from build123d import *

# Parameters (mm, degrees)
SKETCH046_R     = 2.5
PAD023_DEPTH    = 2.5
SKETCH047_R     = 5
PAD024_DEPTH    = 3
FILLET003_R     = 1.5
SKETCH049_R     = 2.5
PAD025_DEPTH    = 4
SKETCH050_R     = 1.5
POCKET026_DEPTH = 4
PAD056_DEPTH    = 0.2


with BuildPart() as part:
    # Sketch046 → Pad023 (new body)
    with BuildSketch(Plane(origin=(0, 0, 30), x_dir=(1, 0, 0), z_dir=(0, 0, -1))):
        with Locations((101, 55)):
            Circle(SKETCH046_R)
    extrude(amount=-PAD023_DEPTH)

    # Sketch047 (on Face3 of Pad023) → Pad024 (join)
    with BuildSketch(Plane.XY.offset(32.5)):
        with Locations((101, -55)):
            Circle(SKETCH047_R)
    extrude(amount=PAD024_DEPTH)

    # Fillet003
    fillet003_edges = [part.edges().sort_by_distance(p)[0] for p in [
        (96, -55, 35.5),
    ]]
    fillet(fillet003_edges, radius=FILLET003_R)

    # Sketch049 → Pad025 (join)
    with BuildSketch(Plane(origin=(0, 0, 30), x_dir=(1, 0, 0), z_dir=(0, 0, -1))):
        with Locations((101, 55)):
            Circle(SKETCH049_R)
    extrude(amount=PAD025_DEPTH)

    # Sketch050 (on Face17 of Pad025) → Pocket026 (cut)
    with BuildSketch(Plane(origin=(0, 0, 26), x_dir=(1, 0, 0), z_dir=(0, 0, -1))):
        with Locations((101, 55)):
            Circle(SKETCH050_R)
    extrude(amount=-POCKET026_DEPTH, mode=Mode.SUBTRACT)


with BuildPart() as part_1:
    # Body002 placement: moved
    add(part.part.moved(Location((75, 0, 0))))

    # Sketch090 (on Face4 of Clone004) → Pad056 (new body)
    with BuildSketch(Plane(origin=(75, 0, 35.5), x_dir=(1, 0, 0), z_dir=(0, 0, 1))):
        Polygon((98.5, -56.5), (103.5, -56.5), (101, -52.5), align=None)
        Polygon((101, -53.5), (99.5, -56), (102.5, -56), align=None, mode=Mode.SUBTRACT)
    extrude(amount=PAD056_DEPTH)


with BuildPart() as part_2:
    # Body013 placement: moved
    add(part_1.part.moved(Location((-52.5, 45, 0))))


solid = part_2.part
Verification items for the finished model (mm, model axes). A direction names the side the tool comes from. Round coordinates to 2 decimals unless told otherwise and drop trailing zeros. Loops run counter-clockwise (first coordinate to the right, second up) from the corner with the lowest first, then second, coordinate; pieces in that order, holes last. Notation, with made-up numbers: (32, 63) - (68, 63) arc R18 cw to (68, 83) - close; hole circle Ø4 at (59.25, 87.25). An arc over 180 degrees is marked (long way). Write item = value, one per line.
Q1. Depth check by flat-ended pin: pin 1 (2 mm diameter, centred on x = 120.5, y = -12.5, fed in from -Z); pin 2 (3 mm diameter, centred on y = -7, z = 34.5, fed in from -X); pin 3 (5 mm diameter, centred on y = -12, z = 29, fed in from +X). Enter the tip coordinate at first touch or a pass-through.
Here are the results:
pin_1 = 32.5
pin_2 = 118.75
pin_3 = 126
Q2. Sectioned sample at A-A on y = -10. Record the boundary of the cut face in (x, z).
Here are the results:
outline = (118.5, 32.5) - (121, 32.5) - (121, 26) - (122, 26) - (122, 30) - (125, 30) - (125, 26) - (126, 26) - (126, 32.5) - (128.5, 32.5) - (128.5, 34) arc R1.5 ccw to (127, 35.5) - (125.06, 35.5) - (125.06, 35.7) - (124.4, 35.7) - (124.4, 35.5) - (122.6, 35.5) - (122.6, 35.7) - (121.94, 35.7) - (121.94, 35.5) - (120, 35.5) arc R1.5 ccw to (118.5, 34) - close
Q3. Sectioned sample at B-B on z = 31.25. Record the boundary of the cut face in (x, y).
Here are the results:
outline = circle Ø5 at (123.5, -10)
Q4. Mould release check, pull along Y, two halves, no side actions. Record for faces 1 (the cylindrical face through (128.119, -11.915, 33.24)), 2 (the flat face through (123, -10, 30)), 3 (the cylindrical face through (122, -10, 28)), 4 (the flat face through (125, -9, 26)): +Y half, -Y half, draft (parallel to the pull), parting line (faces both ways), or undercut.
Here are the results:
face_1 = parting line
face_2 = undercut
face_3 = undercut
face_4 = draft
Q5. Tool access check on faces 5 (the flat face through (124, -9, 35.7)), 6 (the flat face through (121, -11, 32.5)), 7 (the flat face through (123, -10, 35.5)). Record the directions out of +Z, -Z, +X, -X, +Y, -Y that give a thin tool (end or side, any length) a straight path to the whole face; none if there is none.
Here are the results:
face_5 = +Z, +X, -X, +Y, -Y
face_6 = -Z
face_7 = +Z
Q6. Material ranges on L1, parallel to X at y = -10, z = 27.95; L2, parallel to Y at x = 123.5, z = 28.8; L3, parallel to Z at x = 127, y = -10.25, recorded low to high.
Here are the results:
L1 = 121 to 122, 125 to 126
L2 = -12.5 to -11.5, -8.5 to -7.5
L3 = 32.5 to 35.5
Q7. Sectioned sample at C-C on z = 34.25. Record the boundary of the cut face in (x, y), plus the area to 3 significant figures.
Here are the results:
outline = circle Ø9.96 at (123.5, -10)
area = 77.9 mm^2
